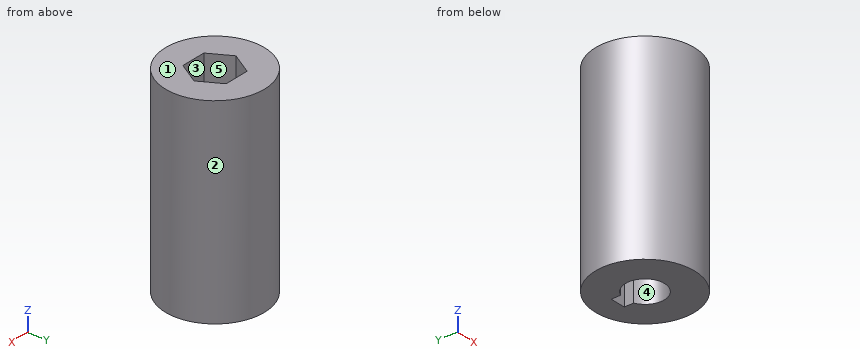
Autodesk Inventor part; units mm, degrees
ref_plane "YZ Plane" through (0, 0, 0) normal (1, 0, 0) x (0, 1, 0)
ref_plane "XZ Plane" through (0, 0, 0) normal (0, 1, 0) x (-1, 0, 0)
ref_plane "XY Plane" through (0, 0, 0) normal (0, 0, 1) x (1, 0, 0)
sketch "Sketch1" plane through (0, 0, 0) normal (0, 0, 1) x (1, 0, 0)
  arc A0 (-1.9939, 4.5894) -> (1.9939, 4.5894) centre (0, 0) ccw
  circle A1 centre (0, 0) radius 12.7
  line L0 (-1.9939, 4.5894) -> (-1.9939, 7.0024)
  line L1 (-1.9939, 7.0024) -> (1.9939, 7.0024)
  line L2 (1.9939, 7.0024) -> (1.9939, 4.5894)
  point P0 (0, 5.0038)
  dimension "d0" = 10.0076
  dimension "d1" = 25.4
  dimension "d5" = 2.413
extrude "Extrusion1" add sketch "Sketch1" along normal blind 25.4
sketch "Sketch2" plane through (0, 0, 25.4) normal (0, 0, 1) x (1, 0, 0)
  line L0 (-1.9939, 4.5894) -> (-1.9939, 7.0024)
  line L1 (-1.9939, 7.0024) -> (1.9939, 7.0024)
  line L2 (1.9939, 7.0024) -> (1.9939, 4.5894)
  arc A0 (-1.9939, 4.5894) -> (1.9939, 4.5894) centre (0, 0) ccw
  circle A1 centre (0, 0) radius 12.7
  circle A2 centre (0, 0) radius 12.7
  line L3 (6.4158, 0) -> (3.2079, -5.5563)
  line L4 (3.2079, -5.5563) -> (-3.2079, -5.5563)
  line L5 (-3.2079, -5.5563) -> (-6.4158, 0)
  line L6 (-6.4158, 0) -> (-3.2079, 5.5562)
  line L7 (-3.2079, 5.5562) -> (3.2079, 5.5563)
  line L8 (3.2079, 5.5563) -> (6.4158, 0)
  line L9 (-1.9939, 7.0024) -> (1.9939, 7.0024)
  line L10 (1.9939, 7.0024) -> (1.9939, 5.5563)
  line L11 (1.9939, 5.5563) -> (-1.9939, 5.5563)
  line L12 (-1.9939, 5.5563) -> (-1.9939, 7.0024)
  dimension "d8" = 11.1125
extrude "Extrusion2" add sketch "Sketch2" along normal blind 25.4 contours L0 L1 L2 L7 | A1
properties material "ABS Plastic"
Check sheet for the modelled part. Datum: model origin and axes. Units: mm. Face numbers are marked on the shaded views. A direction names the side the tool comes from. Give positions to 0.01 mm unless a question says otherwise; leave off trailing zeros. Loops run counter-clockwise (first coordinate to the right, second up) from the corner with the lowest first, then second, coordinate; pieces in that order, holes last. Notation, with made-up numbers: M 76,26 L 80,26 A10 ccw 80,39 Z; hole C 28,-32 d5. An arc over 180 degrees is marked long. Answer in a Markdown table with one row per item.
1) Thickness scan on line 1 (Y direction, x = 0, z = 9.5); line 2 (X direction, y = -1, z = 27); line 3 (X direction, y = 4.5, z = 11.5). Record the ranges inside material, lowest first.
Solutions:
| item | result |
|---|---|
| line 1 | y = -12.7 to -5, 7 to 12.7 |
| line 2 | x = -12.66 to -5.84, 5.84 to 12.66 |
| line 3 | x = -11.88 to -2.19, 2.19 to 11.88 |
2) Depth check by flat-ended pin: pin 1 (5 mm diameter, centred on x = 4, y = -9, fed in from -Z); pin 2 (4 mm diameter, centred on y = -3, z = 21, fed in from -X); pin 3 (1.9 mm diameter, centred on y = 5.5, z = 7, fed in from +X); pin 4 (1.2 mm diameter, centred on y = 5, z = 16, fed in from -X). Enter the tip coordinate at first touch or a pass-through.
Solutions:
| item | result |
|---|---|
| pin 1 | stops at z = 0 |
| pin 2 | stops at x = -12.66 |
| pin 3 | stops at x = 11.86 |
| pin 4 | stops at x = -11.91 |
3) Cross-section at B-B (x = 4). Enter the section's corners in (y, z), plus the area to 3 significant figures.
Solutions:
| item | result |
|---|---|
| outline | M -12.05,0 L -3.01,0 L -3.01,25.4 L -4.18,25.4 L -4.18,50.8 L -12.05,50.8 Z; M 3.01,0 L 12.05,0 L 12.05,50.8 L 4.18,50.8 L 4.18,25.4 L 3.01,25.4 Z |
| area | 859 mm^2 |
4) Tool access check on the marked faces 4 and 5. Record the directions out of +Z, -Z, +X, -X, +Y, -Y that give a thin tool (end or side, any length) a straight path to the whole face; none if there is none.
Solutions:
| item | result |
|---|---|
| face 4 | +Z, -Z |
| face 5 | +Z |
5) Cross-section at C-C (z = 23). Enter the section's corners in (x, y), plus the area to 3 significant figures.
Solutions:
| item | result |
|---|---|
| outline | C 0,0 d25.4; hole M -1.99,4.59 A5 ccw long 1.99,4.59 L 1.99,7 L -1.99,7 Z |
| area | 420 mm^2 |
6) Cross-section at D-D (x = 0). Enter the section's corners in (y, z).
Solutions:
| item | result |
|---|---|
| outline | M -12.7,0 L -5,0 L -5,25.4 L -5.56,25.4 L -5.56,50.8 L -12.7,50.8 Z; M 5.56,25.4 L 7,25.4 L 7,0 L 12.7,0 L 12.7,50.8 L 5.56,50.8 Z |
7) Cross-section at A-A (z = 38.5). Enter the section's corners in (x, y).
Solutions:
| item | result |
|---|---|
| outline | C 0,0 d25.4; hole M -6.42,0 L -3.21,-5.56 L 3.21,-5.56 L 6.42,0 L 3.21,5.56 L -3.21,5.56 Z |
8) Mould release check, pull along Y, two halves, no side actions. Record for the marked faces 1, 2 and 3: released by +Y, released by -Y, zero draft, split by the parting line, or undercut.
Solutions:
| item | result |
|---|---|
| face 1 | zero draft |
| face 2 | split by the parting line |
| face 3 | undercut |
